The listing builds one solid part. Answer for the finished solid, in the listing's coordinates (mm). Give positions to 0.01 mm unless a question says otherwise; leave off trailing zeros. Write each loop counter-clockwise with the first axis right and the second up, starting at its lowest first coordinate (ties: lowest second). Pieces come first, ordered by that corner, then holes. Notation, with made-up numbers: (10.25, 85.5) - (65.25, 85.5) arc R18 cw to (65.25, 102.5) - close; hole circle Ø3 at (-11.75, 11). An arc over 180 degrees is marked (long way). Return JSON: item names as keys, results as strings.
from build123d import *

# Parameters (mm, degrees)
CROQUIS1_R              = 35
CROQUIS1_R_2            = 12.5
CROQUIS1_R_3            = 1.5
SALIENTE_EXTRUIR1_DEPTH = 3
REDONDEO1_R             = 1


with BuildPart() as part:
    # Croquis1 → Saliente-Extruir1 (new body)
    with BuildSketch(Plane.XY):
        Circle(CROQUIS1_R)
        Circle(CROQUIS1_R_2, mode=Mode.SUBTRACT)
        with Locations((30, 0)):
            Circle(CROQUIS1_R_3, mode=Mode.SUBTRACT)
        with Locations((-30, 0)):
            Circle(CROQUIS1_R_3, mode=Mode.SUBTRACT)
    extrude(amount=SALIENTE_EXTRUIR1_DEPTH)

    # Redondeo1
    redondeo1_edges = [part.edges().sort_by_distance(p)[0] for p in [
        (-35, 0, 0),
        (-35, 0, 3),
        (-12.5, 0, 0),
        (-12.5, 0, 3),
    ]]
    fillet(redondeo1_edges, radius=REDONDEO1_R)


solid = part.part
Item 1: A cutting plane is placed at A-A on y = 0. Determine the outline of the cut face in (x, z).
Answer below:
{"outline": "(-35, 1) arc R1 ccw to (-34, 0) - (-31.5, 0) - (-31.5, 3) - (-34, 3) arc R1 ccw to (-35, 2) - close; (-28.5, 0) - (-13.5, 0) arc R1 ccw to (-12.5, 1) - (-12.5, 2) arc R1 ccw to (-13.5, 3) - (-28.5, 3) - close; (12.5, 1) arc R1 ccw to (13.5, 0) - (28.5, 0) - (28.5, 3) - (13.5, 3) arc R1 ccw to (12.5, 2) - close; (31.5, 0) - (34, 0) arc R1 ccw to (35, 1) - (35, 2) arc R1 ccw to (34, 3) - (31.5, 3) - close"}
Item 2: A cutting plane is placed at B-B on x = 0. Determine the outline of the cut face in (y, z), then the cut area to 3 significant figures.
Answer below:
{"outline": "(-35, 1) arc R1 ccw to (-34, 0) - (-13.5, 0) arc R1 ccw to (-12.5, 1) - (-12.5, 2) arc R1 ccw to (-13.5, 3) - (-34, 3) arc R1 ccw to (-35, 2) - close; (12.5, 1) arc R1 ccw to (13.5, 0) - (34, 0) arc R1 ccw to (35, 1) - (35, 2) arc R1 ccw to (34, 3) - (13.5, 3) arc R1 ccw to (12.5, 2) - close", "area": "133 mm²"}
Item 3: The mould has two halves that part along X. Classify faces 1 (the face through (-27.77, -21.3, 1.49)), 2 (the face through (-31.5, 0.07, 1.48)), 3 (the face through (15, 0, 0)): +X half, -X half, draft (parallel to the pull), parting line (faces both ways), or undercut.
Answer below:
{"face 1": "parting line", "face 2": "undercut", "face 3": "draft"}
Item 4: Consider L1, parallel to Y at x = -30, z = 1.5; L2, parallel to Y at x = 29.5, z = 2.3; L3, parallel to X at y = 5.5, z = 1.35. Determine where each line is inside the solid, lowest interval first.
Answer below:
{"L1": "y = -18.03 to -1.5, 1.5 to 18.03", "L2": "y = -18.75 to -1.41, 1.41 to 18.75", "L3": "x = -34.57 to -11.22, 11.22 to 34.57"}
Item 5: Flat-ended cylindrical pins translate along their axes: P1, Ø2.5, axis at x = 30, y = 0, coming from the +Z side; P2, Ø1, axis at y = 19, z = 2.5, coming from the -X side; P3, Ø1, axis at y = 2.5, z = 1.5, coming from the -X side; P4, Ø1, axis at y = -27.5, z = 2.5, coming from the -X side. Find the tip coordinate at first contact, or state that the pin passes through.
Answer below:
{"P1": "passes through", "P2": "stops at x = -29.63", "P3": "stops at x = -34.94", "P4": "stops at x = -22.15"}
